Work out the finished part from the listing and answer in its coordinate system (mm). Round coordinates to 2 decimals unless told otherwise and drop trailing zeros. Write each loop counter-clockwise with the first axis right and the second up, starting at its lowest first coordinate (ties: lowest second). Pieces come first, ordered by that corner, then holes.
1. Straight lines are drawn through the part: probe 1 along Z at (x, y) = (3.55, 9); probe 2 along Y at (x, z) = (1.2, -41); probe 3 along Y at (x, z) = (0.2, -7). For each, find the intervals that lie inside material, in ascending order.
2. Find section C-C (z = -26). Write down the section's boundary in (x, y), and give its area (3 significant figures).
3. Find section D-D (y = 17). Write down the section's boundary in (x, z) (3 decimals), and give its area (3 significant figures).
```python
from build123d import *

# Parameters (mm, degrees)
BOSS_EXTRUDE1_DEPTH = 3.77
FILLET1_R           = 0.2
CAVITY1_DEPTH       = 32.53
CUT_EXTRUDE1_DEPTH  = 10


# Read off the part's stored shape, not the designer's step: Cavity1
with BuildPart() as part:
    # Sketch1 → Boss-Extrude1 (new body)
    with BuildSketch(Plane(origin=(0, 0, 0), x_dir=(0, 0, -1), z_dir=(1, 0, 0))):
        Polygon((0, 0), (60, 0), (0, 32.53), align=None)
    extrude(amount=BOSS_EXTRUDE1_DEPTH)

    # Fillet1
    fillet1_edges = [part.edges().sort_by_distance(p)[0] for p in [
        (1.885, 0, -60),
    ]]
    fillet(fillet1_edges, radius=FILLET1_R)

    # Cavity1 outline → Cavity1 (cut)
    with BuildSketch(Plane(origin=(0, 0, 0), x_dir=(1, 0, 0), z_dir=(0, 1, 0))):
        with BuildLine():
            Line((3.77, 0), (3.77, 3.2038331))
            ThreePointArc((3.77, 3.2038331), (1.741729711, 1.914090145), (0, 0.257679909))
            Line((0, 0.257679909), (0, 0))
            Line((0, 0), (3.77, 0))
        make_face()
    extrude(amount=CAVITY1_DEPTH, mode=Mode.SUBTRACT)

    # Sketch2 → Cut-Extrude1 (cut)
    with BuildSketch(Plane.ZY):
        Polygon((-46.188988267, 0), (-46.188988267, 7.48784154), (-59.313137704, 0.37224377), (-59.211490846, 0), align=None)
    extrude(amount=-CUT_EXTRUDE1_DEPTH, mode=Mode.SUBTRACT)


with BuildPart() as cut_extrude1_kept_piece:
    # of the separate pieces the step leaves, the one the design keeps (cut_extrude1_pieces_kept)
    add(part.part.solids().sort_by_distance((0, 0, -0.257679909))[0])


solid = cut_extrude1_kept_piece.part
```
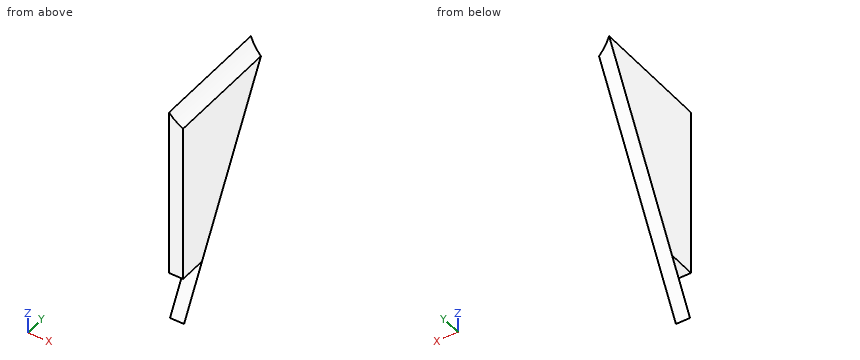
Worked answers:
1. probe 1: z = -43.4 to -3.09
1. probe 2: y = 0 to 10.3
1. probe 3: y = 0 to 28.73
2. outline: (0, 0) - (3.77, 0) - (3.77, 18.43) - (0, 18.43) - close
2. area: 69.5 mm2
3. outline: (0, -28.644) - (3.77, -28.644) - (3.77, -3.204) arc R12.415 cw to (0, -0.258) - close
3. area: 101 mm2
